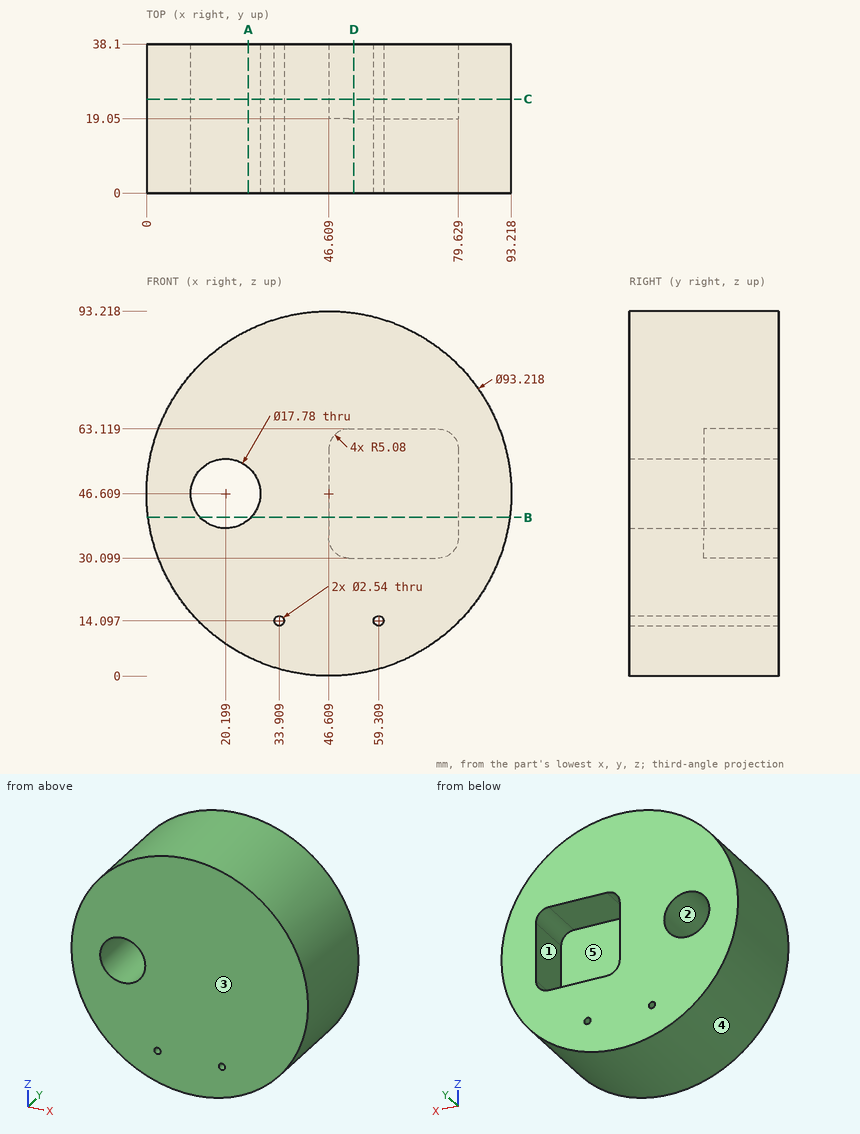
Can you work these out from the drawing? Everything is in mm from the part's minimum corner. A direction names the side the tool comes from. Round coordinates to 2 decimals unless told otherwise and drop trailing zeros. Write each loop counter-clockwise with the first axis right and the second up, starting at its lowest first coordinate (ties: lowest second). Pieces come first, ordered by that corner, then holes.
1. Will these pins go through, and if not, where does the flat tip stop? pin 1 Ø3.5 at (x, z) = (59.309, 14.097) entering from +Y; pin 2 Ø2 at (x, y) = (32, 10.5) entering from -Z; pin 3 Ø8 at (y, z) = (9, 68) entering from +X; pin 4 Ø6 at (x, y) = (72.5, 20) entering from -Z.
2. Suppose I cut it at B-B (z = 40.5). List the corners of the cut face in (x, y) for me, and give its area (3 significant figures).
3. I need wall thicknesses on L1, parallel to X at y = 20, z = 47.5; L2, parallel to X at y = 20, z = 14.5; L3, parallel to X at y = 9.5, z = 45. Which ranges of each line are inside material? Lowest first, please.
4. Suppose I cut it at C-C (y = 24). List the corners of the cut face in (x, z) for me.
5. For the marked faces 1 and 2, which set-ups out of +Z, -Z, +X, -X, +Y, -Y let a thin tool reach every point of the face, with its end or its side?
6. Suppose I cut it at D-D (x = 53). List the corners of the cut face in (y, z) for me.
7. Suppose I cut it at A-A (x = 26). List the corners of the cut face in (y, z) for me.
8. If we mould it in two halves opening along X, with no side actions, what happens to the marked faces 3, 4 and 5? For each: released by +X, released by -X, zero draft, split by the parting line, or undercut.
Answer sheet:
1. pin 1: stops at y = 38.1
1. pin 2: stops at z = 2.03
1. pin 3: stops at x = 89.85
1. pin 4: stops at z = 6.01
2. outline: (0.4, 0) - (13.74, 0) - (13.74, 38.1) - (0.4, 38.1) - close; (26.66, 0) - (92.82, 0) - (92.82, 38.1) - (79.63, 38.1) - (79.63, 19.05) - (46.61, 19.05) - (46.61, 38.1) - (26.66, 38.1) - close
2. area: 2,400 mm2
3. L1: x = 0.01 to 11.35, 29.04 to 46.61, 79.63 to 93.21
3. L2: x = 12.82 to 32.7, 35.11 to 58.1, 60.51 to 80.39
3. L3: x = 0.03 to 11.46, 28.94 to 93.19
4. outline: circle Ø93.22 at (46.61, 46.61); hole circle Ø17.78 at (20.2, 46.61); hole circle Ø2.54 at (33.91, 14.1); hole (46.61, 35.18) arc R5.08 ccw to (51.69, 30.1) - (74.55, 30.1) arc R5.08 ccw to (79.63, 35.18) - (79.63, 58.04) arc R5.08 ccw to (74.55, 63.12) - (51.69, 63.12) arc R5.08 ccw to (46.61, 58.04) - close; hole circle Ø2.54 at (59.31, 14.1)
5. face 1: +Y
5. face 2: +Y, -Y
6. outline: (0, 0.44) - (38.1, 0.44) - (38.1, 30.1) - (19.05, 30.1) - (19.05, 63.12) - (38.1, 63.12) - (38.1, 92.78) - (0, 92.78) - close
7. outline: (0, 4.8) - (38.1, 4.8) - (38.1, 39.87) - (0, 39.87) - close; (0, 53.35) - (38.1, 53.35) - (38.1, 88.41) - (0, 88.41) - close
8. face 3: zero draft
8. face 4: split by the parting line
8. face 5: undercut
